from build123d import *

# Parameters (mm, degrees)
F0_W          = 76.57
F0_H          = 136.35
F0_R          = 1.7272
F1_DEPTH      = 24
F2_R          = 12.7
F3_DEPTH      = 8.47
F3_DEPTH_BACK = 40
F5_DEPTH      = 26
F6_W          = 66.04
F6_H          = 76.2
F7_DEPTH      = 76.2
F8_R          = 82.55
F9_DEPTH      = 38.1
F10_R         = 10


with BuildPart() as f1:
    # F0 (on Top) → F1 (new body)
    with BuildSketch(Plane.XY):
        Rectangle(F0_W, F0_H)
        with Locations((-30, -63.175)):
            Circle(F0_R, mode=Mode.SUBTRACT)
        with Locations((-30, -3.175)):
            Circle(F0_R, mode=Mode.SUBTRACT)
        with Locations((30, -63.175)):
            Circle(F0_R, mode=Mode.SUBTRACT)
        with Locations((30, -3.175)):
            Circle(F0_R, mode=Mode.SUBTRACT)
    extrude(amount=F1_DEPTH)

    # F2 (on face) → F3 (join, two sides)
    with BuildSketch(Plane.XY.offset(24)) as f3_sk:
        with Locations((0, -33.175)):
            Circle(F2_R)
    extrude(amount=F3_DEPTH)
    extrude(f3_sk.sketch, amount=-F3_DEPTH_BACK)

    # F4 (on face) → F5 (join)
    with BuildSketch(Plane.XY.offset(32.47)):
        with BuildLine():
            ThreePointArc((-3.714835, -28.025), (0, -39.525), (3.714835, -28.025))
            Line((3.714835, -28.025), (-3.714835, -28.025))
        make_face()
    extrude(amount=F5_DEPTH)

    # F6 (on face) → F7 (join)
    with BuildSketch(Plane(origin=(0, 0, 0), x_dir=(1, 0, 0), z_dir=(0, 0, -1))):
        with Locations((0, -23.979)):
            Rectangle(F6_W, F6_H)
    extrude(amount=F7_DEPTH)

    # F8 (on face) → F9 (join)
    with BuildSketch(Plane(origin=(0, 0, -76.2), x_dir=(1, 0, 0), z_dir=(0, 0, -1))):
        with Locations((0, -43.029)):
            Circle(F8_R)
    extrude(amount=F9_DEPTH)

    # F10
    f10_edges = [f1.edges().sort_by_distance(p)[0] for p in [
        (-33.02, 62.079, -38.1),
        (-33.02, -14.121, -38.1),
        (33.02, 62.079, -38.1),
        (33.02, -14.121, -38.1),
        (38.285, 68.175, 12),
        (-38.285, 68.175, 12),
        (-38.285, -68.175, 12),
        (38.285, -68.175, 12),
    ]]
    fillet(f10_edges, radius=F10_R)


solid = f1.part
Can you work these out from the model? Positions are in its coordinate system, mm. A direction names the side the tool comes from. Round coordinates to 2 decimals unless told otherwise and drop trailing zeros. Write each loop counter-clockwise with the first axis right and the second up, starting at its lowest first coordinate (ties: lowest second). Pieces come first, ordered by that corner, then holes. Notation, with made-up numbers: M -17,54 L 42,54 A14 cw 42,68 Z; hole C 66,34 d8. An arc over 180 degrees is marked long. Use a Markdown table: item, result.
Item 1: For pin 1 Ø23 at (x, z) = (-2, -30.5) entering from -Y; pin 2 Ø7 at (y, z) = (1.5, 6.5) entering from -X (3 decimals); pin 3 Ø17 at (y, z) = (18.5, -40) entering from -X, each with a flat end and sliding along its axis, tell me the tip position at first contact or that it passes through.
Found:
| item | result |
|---|---|
| pin 1 | stops at y = -14.12 |
| pin 2 | stops at x = -38.285 |
| pin 3 | stops at x = -33.02 |
Item 2: I want a section at A-A (z = -11). List the corners of the cut face in (x, y) for me (3 decimals).
Found:
| item | result |
|---|---|
| outline | M -33.02,-4.121 A10 ccw -23.02,-14.121 L 23.02,-14.121 A10 ccw 33.02,-4.121 L 33.02,52.079 A10 ccw 23.02,62.079 L -23.02,62.079 A10 ccw -33.02,52.079 Z; C 0,-33.175 d25.4 |
Item 3: If I drill on line 1 along Y through (x, z) = (-30, 5); line 2 along X through (y, z) = (-45, 13) (3 decimals); line 3 along Z through (x, y) = (-41.5, 69), over which ranges is the centre line in solid material (lowest first)? Write a range as [from, to].
Found:
| item | result |
|---|---|
| line 1 | y = [-68.03, -64.9], [-61.45, -4.9], [-1.45, 68.03] |
| line 2 | x = [-38.285, 38.285] |
| line 3 | z = [-114.3, -76.2] |
Item 4: I want a section at C-C (y = -9.5). List the corners of the cut face in (x, z) for me (1 decimal), and give its area (3 significant figures).
Found:
| item | result |
|---|---|
| outline | M -63.7,-114.3 L 63.7,-114.3 L 63.7,-76.2 L 31.5,-76.2 L 31.5,0 L 38.3,0 L 38.3,24 L -38.3,24 L -38.3,0 L -31.5,0 L -31.5,-76.2 L -63.7,-76.2 Z |
| area | 11,500 mm2 |
Item 5: I want a section at D-D (z = -84.5). List the corners of the cut face in (x, y) for me.
Found:
| item | result |
|---|---|
| outline | C 0,43.03 d165.1 |
Item 6: I want a section at B-B (x = 0). List the corners of the cut face in (y, z) for me (3 decimals).
Found:
| item | result |
|---|---|
| outline | M -68.175,0 L -45.875,0 L -45.875,-16 L -20.475,-16 L -20.475,0 L -14.121,0 L -14.121,-76.2 L -39.521,-76.2 L -39.521,-114.3 L 125.579,-114.3 L 125.579,-76.2 L 62.079,-76.2 L 62.079,0 L 68.175,0 L 68.175,24 L -20.475,24 L -20.475,32.47 L -28.025,32.47 L -28.025,58.47 L -39.525,58.47 L -39.525,32.47 L -45.875,32.47 L -45.875,24 L -68.175,24 Z |
Item 7: Which directions (+Z, -Z, +X, -X, +Y, -Y) give clear straight access to the entire face, cutting with the end or side of a thin tool? Please do faces 4 (the face through (0, -27, 32.47)), 5 (the face through (0, -28.025, 45)), 6 (the face through (33.02, 24, -38)), 7 (the face through (0, -14.121, -38)), 8 (the face through (0, 62.079, -38)).
Found:
| item | result |
|---|---|
| face 4 | +Z |
| face 5 | +Z, +X, -X, +Y |
| face 6 | +X, +Y, -Y |
| face 7 | +X, -X |
| face 8 | +X, -X, +Y |
Item 8: We'd pull the mould along Y, two halves only. Please class faces 1 (the face through (-33.02, 24, -38)), 2 (the face through (5.86, -44.44, -7.89)), 3 (the face through (-0.22, -39.52, 45.29)): released by +Y, released by -Y, zero draft, split by the parting line, or undercut.
Found:
| item | result |
|---|---|
| face 1 | zero draft |
| face 2 | undercut |
| face 3 | split by the parting line |
